The listing builds one solid part. Answer for the finished solid, in the listing's coordinates (mm). Coordinates: 2 decimals unless noted, no trailing zeros. Order: outer loops, then holes, each group sorted by start corner. A loop starts at its lowest first (then second) coordinate and runs counter-clockwise, first axis right, second up.
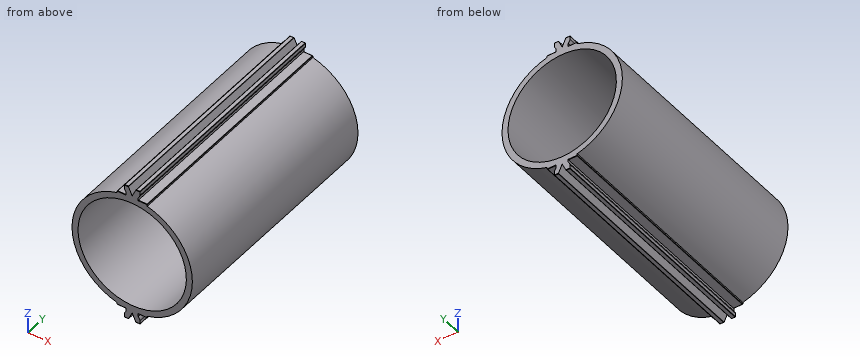
```python
from build123d import *

# Parameters (mm, degrees)
SKETCH_1_R             = 15
SKETCH_1_R_2           = 13.5
EXTRUDE_1_DEPTH        = 58
EXTRUDE_2_DEPTH        = 58
EXTRUDE_3_DEPTH        = 58
FILLET_1_R             = 0.1
MIRROR_2_COPY_1_DEPTH  = 58
FILLET_1_OF_MIRROR_2_R = 0.1


with BuildPart() as part:
    # 草图1 → 凸台-拉伸1 (new body)
    with BuildSketch(Plane(origin=(0, 0, 0), x_dir=(1, 0, 0), z_dir=(0, 1, 0))):
        with Locations(Location((0, 0, 0), (0, 0, 90))):
            Circle(SKETCH_1_R)
        with Locations(Location((0, 0, 0), (0, 0, 90))):
            Circle(SKETCH_1_R_2, mode=Mode.SUBTRACT)
    extrude(amount=EXTRUDE_1_DEPTH)

    # 草图10 → 凸台-拉伸2 (add)
    with BuildSketch(Plane(origin=(0, 0, 0), x_dir=(1, 0, 0), z_dir=(0, 1, 0))):
        with BuildLine():
            Line((0, 15), (3.75, 15))
            Line((3.75, 15), (3.75, 14.523687548))
            ThreePointArc((3.75, 14.523687548), (1.890064387, 14.880445444), (0, 15))
        make_face()
    extrude_2 = extrude(amount=EXTRUDE_2_DEPTH)

    # 镜向1: 凸台-拉伸2 across plane
    add(extrude_2.mirror(Plane(origin=(0, 0, 0), x_dir=(0, 0, 1), z_dir=(1, 0, 0))))

    # 草图11 → 凸台-拉伸3 (add)
    with BuildSketch(Plane(origin=(0, 0, 0), x_dir=(1, 0, 0), z_dir=(0, 1, 0))):
        with BuildLine():
            Line((-1.5, 15), (1.5, 15))
            Line((1.5, 15), (1.5, 15.677124344))
            ThreePointArc((1.5, 15.677124344), (1.780042303, 16.088161527), (1.95, 16.555590279))
            Line((1.95, 16.555590279), (1.95, 17.5))
            Line((1.95, 17.5), (0.95, 17.5))
            Line((0.95, 17.5), (0, 15.462718426))
            Line((0, 15.462718426), (-0.95, 17.5))
            Line((-0.95, 17.5), (-1.95, 17.5))
            Line((-1.95, 17.5), (-1.95, 16.555590279))
            ThreePointArc((-1.95, 16.555590279), (-1.780042303, 16.088161527), (-1.5, 15.677124344))
            Line((-1.5, 15.677124344), (-1.5, 15))
        make_face()
    extrude_3 = extrude(amount=EXTRUDE_3_DEPTH)

    # 圆角1
    fillet_1_edges = [part.edges().sort_by_distance(p)[0] for p in [
        (-0.95, 29, -17.5),
        (-1.45, 58, -17.5),
        (-1.95, 29, -17.5),
        (-1.45, 0, -17.5),
        (1.95, 29, -17.5),
        (1.45, 58, -17.5),
        (0.95, 29, -17.5),
        (1.45, 0, -17.5),
        (-2.625, 58, -15),
        (-2.625, 0, -15),
        (2.625, 58, -15),
        (2.625, 0, -15),
        (3.75, 29, -15),
        (-3.75, 29, -15),
    ]]
    fillet(fillet_1_edges, radius=FILLET_1_R)

    # 镜向2: 凸台-拉伸2, 凸台-拉伸3 across plane
    add(extrude_2.mirror(Plane.XY))
    add(extrude_3.mirror(Plane.XY))

    # 镜向2 copy 1 sketch → 镜向2 copy 1 (add)
    with BuildSketch(Plane(origin=(0, 0, 0), x_dir=(-1, 0, 0), z_dir=(0, 1, 0))):
        with BuildLine():
            Line((0, 15), (3.75, 15))
            Line((3.75, 15), (3.75, 14.523687548))
            ThreePointArc((3.75, 14.523687548), (1.890064387, 14.880445444), (0, 15))
        make_face()
    extrude(amount=MIRROR_2_COPY_1_DEPTH)

    # 圆角1 of 镜向2
    fillet_1_of_mirror_2_edges = [part.edges().sort_by_distance(p)[0] for p in [
        (-0.95, 29, 17.5),
        (-1.45, 58, 17.5),
        (-1.95, 29, 17.5),
        (-1.45, 0, 17.5),
        (1.95, 29, 17.5),
        (1.45, 58, 17.5),
        (0.95, 29, 17.5),
        (1.45, 0, 17.5),
        (-2.625, 58, 15),
        (-2.625, 0, 15),
        (2.625, 58, 15),
        (2.625, 0, 15),
        (3.75, 29, 15),
        (-3.75, 29, 15),
    ]]
    fillet(fillet_1_of_mirror_2_edges, radius=FILLET_1_OF_MIRROR_2_R)


solid = part.part
```
(1) Find section B-B (x = -7.75). Write down the section's boundary in (y, z), and give its area (3 significant figures).
(2) Find section C-C (x = 2.75). Write down the section's boundary in (y, z).
(3) Consider line 1 (Z direction, x = 11, y = 20); line 2 (Z direction, x = -9, y = 17); line 3 (X direction, y = 53.5, z = 10). Determine where each line is inside the solid, lowest interval first.
(4) Find section A-A (z = 0). Write down the section's boundary in (x, y), and give its area (3 significant figures).
(5) Each of these flat-tipped pins is pushed along its axis until it touches: pin 1 Ø4 at (x, y) = (-7, 34.5) entering from -Z; pin 2 Ø3 at (y, z) = (6, 4.5) entering from +X; pin 3 Ø1.5 at (y, z) = (6, 4.5) entering from -X; pin 4 Ø3 at (x, z) = (5, 10) entering from +Y. Where does it stop, or does it pass through?
Findings below:
1. outline: (0, -12.84) - (58, -12.84) - (58, -11.05) - (0, -11.05) - close; (0, 11.05) - (58, 11.05) - (58, 12.84) - (0, 12.84) - close
1. area: 208 mm2
2. outline: (0, -14.9) arc R0.1 ccw to (0.1, -15) - (57.9, -15) arc R0.1 ccw to (58, -14.9) - (58, -13.22) - (0, -13.22) - close; (0, 13.22) - (58, 13.22) - (58, 14.9) arc R0.1 ccw to (57.9, 15) - (0.1, 15) arc R0.1 ccw to (0, 14.9) - close
3. line 1: z = -10.2 to -7.83, 7.83 to 10.2
3. line 2: z = -12 to -10.06, 10.06 to 12
3. line 3: x = -11.18 to -9.07, 9.07 to 11.18
4. outline: (-15, 0) - (-13.5, 0) - (-13.5, 58) - (-15, 58) - close; (13.5, 0) - (15, 0) - (15, 58) - (13.5, 58) - close
4. area: 174 mm2
5. pin 1: stops at z = -14.14
5. pin 2: stops at x = 14.7
5. pin 3: stops at x = -14.52
5. pin 4: passes through
